from build123d import *

# Parameters (mm, degrees)
SKETCH_1_W             = 30
SKETCH_1_H             = 20
SKETCH_1_R             = 3.5
EXTRUDE_1_DEPTH        = 15
HOLE_WIZARD_M6_1_D     = 5
HOLE_WIZARD_M6_1_DEPTH = 15
HOLE_WIZARD_M6_1_TIP   = 1.502151548


with BuildPart() as part:
    # 草图1 → 凸台-拉伸1 (new body)
    with BuildSketch(Plane.XY):
        Rectangle(SKETCH_1_W, SKETCH_1_H)
        with Locations((-7.5, 0)):
            Circle(SKETCH_1_R, mode=Mode.SUBTRACT)
        with Locations((7.5, 0)):
            Circle(SKETCH_1_R, mode=Mode.SUBTRACT)
    extrude(amount=EXTRUDE_1_DEPTH)

    # M6 螺纹孔1
    with Locations(Plane(origin=(0, 10, 7.5), x_dir=(0, 0, 1), z_dir=(0, 1, 0))):
        with Locations((0, 0)):
            Hole(HOLE_WIZARD_M6_1_D / 2, depth=HOLE_WIZARD_M6_1_DEPTH)
            with Locations((0, 0, -(HOLE_WIZARD_M6_1_DEPTH + HOLE_WIZARD_M6_1_TIP / 2))):  # 118° drill point
                Cone(0, HOLE_WIZARD_M6_1_D / 2, HOLE_WIZARD_M6_1_TIP, mode=Mode.SUBTRACT)


solid = part.part
Geometry: final body of the model. Coordinates: model frame, mm. A direction names the side the tool comes from. Round coordinates to 2 decimals unless told otherwise and drop trailing zeros. Order: outer loops, then holes, each group sorted by start corner. A loop starts at its lowest first (then second) coordinate and runs counter-clockwise, first axis right, second up.
Q1. Section D-D, the plane y = 8.25. Output: boundary loops of the cut face in (x, z).
Result sheet:
outline: (-15, 0) - (15, 0) - (15, 15) - (-15, 15) - close; hole circle Ø5 at (0, 7.5)
Q2. Section B-B, the plane x = -7.5. Output: boundary loops of the cut face in (y, z).
Result sheet:
outline: (-10, 0) - (-3.5, 0) - (-3.5, 15) - (-10, 15) - close; (3.5, 0) - (10, 0) - (10, 15) - (3.5, 15) - close
Q3. Mould query, pull axis Y, two halves, no side actions, for faces 3 (the face through (-11, 0, 7)), 4 (the face through (15, 0, 7)), 5 (the face through (0.019, -6.241, 7.066)). Classes: released by +Y, released by -Y, zero draft, split by the parting line, or undercut.
Result sheet:
face 3: undercut
face 4: zero draft
face 5: released by +Y
Q4. Section A-A, the plane y = 0. Output: boundary loops of the cut face in (x, z).
Result sheet:
outline: (-15, 0) - (-11, 0) - (-11, 15) - (-15, 15) - close; (-4, 0) - (4, 0) - (4, 15) - (-4, 15) - close; (11, 0) - (15, 0) - (15, 15) - (11, 15) - close; hole circle Ø5 at (0, 7.5)
Q5. Material intervals for probe 1 along X at (y, z) = (4.5, 7.5); probe 2 along Z at (x, y) = (0, 2.25); probe 3 along X at (y, z) = (-0.5, 9.25), sorted ascending.
Result sheet:
probe 1: x = -15 to -2.5, 2.5 to 15
probe 2: z = 0 to 5, 10 to 15
probe 3: x = -15 to -10.96, -4.04 to -1.79, 1.79 to 4.04, 10.96 to 15
Q6. Pin query (flat end, axial travel): pin 1 (9 mm diameter, centred on x = -7.5, y = 0, fed in from -Z); pin 2 (5.5 mm diameter, centred on x = 7.5, y = 0, fed in from -Z) (3 decimals). Return the tip coordinate at first contact, or that it passes through.
Result sheet:
pin 1: stops at z = 0
pin 2: passes through
Q7. Section C-C, the plane z = 10.5. Output: boundary loops of the cut face in (x, y), and give its area (3 significant figures).
Result sheet:
outline: (-15, -10) - (15, -10) - (15, 10) - (-15, 10) - close; hole circle Ø7 at (-7.5, 0); hole circle Ø7 at (7.5, 0)
area: 523 mm2
Q8. Access query for faces 1 (the face through (0, 2, 10)), 2 (the face through (-4, 10, 7)). Directions: +Z, -Z, +X, -X, +Y, -Y. A direction counts if a zero-diameter tool reaches every point of the face in a straight line with its end or side. Return the directions, or none.
Result sheet:
face 1: +Y
face 2: +Z, -Z, +X, -X, +Y
